Check sheet for the modelled part. Datum: model origin and axes. Units: mm. A direction names the side the tool comes from. Coordinates: 2 decimals unless noted, no trailing zeros. Order: outer loops, then holes, each group sorted by start corner. A loop starts at its lowest first (then second) coordinate and runs counter-clockwise, first axis right, second up.
1. Set-up check for faces 1 (the cylindrical face through (-12.71, -0.95, 3.03)), 2 (the cylindrical face through (0.13, 1.72, -5.45)), 3 (the flat face through (9.525, 2.4, -2.4)): record each of +Z, -Z, +X, -X, +Y, -Y from which the full face is reachable in a straight line by a thin tool's end or side.
2. Thickness scan on line 1 (Y direction, x = 2, z = 0) (3 decimals); line 2 (Z direction, x = 11, y = 0.75); line 3 (Z direction, x = 9, y = -1.25). Record the ranges inside material, lowest first.
3. Cross-section at C-C (x = -12). Enter the section's corners in (y, z) (3 decimals).
4. Draft check along Y on faces 4 (the flat face through (-9.525, 2.4, -2.4)), 5 (the cylindrical face through (-0.221, 0.607, 1.926)), 6 (the cylindrical face through (12.71, -0.95, 3.03)). Enter one of: released by +Y, released by -Y, zero draft, split by the parting line, or undercut.
5. Gauge pin test, flat ends, axial feed: pin 1 Ø2 at (y, z) = (4.5, 1.5) entering from -X (3 decimals); pin 2 Ø4 at (x, z) = (-2.5, 3.5) entering from -Y; pin 3 Ø1 at (x, z) = (-2, -1) entering from +Y. Record the tip position at first contact, or that the pin passes through.
```python
from build123d import *

# Parameters (mm, degrees)
SKETCH34_R                  = 5.715
BOSS_EXTRUDE2_DEPTH         = 15.875
F_21_0_159_DIAMETER_HOLE2_D = 4.0386
SKETCH39_W                  = 6.35
SKETCH39_H                  = 2.54
CHAMFER1_SIZE               = 0.0762
CHAMFER2_SIZE               = 0.0762
CHAMFER8_SIZE               = 0.0762


with BuildPart() as part:
    # Sketch34 → Boss-Extrude2 (new, symmetric)
    with BuildSketch(Plane(origin=(0, 0, 0), x_dir=(0, 0, -1), z_dir=(1, 0, 0))):
        Circle(SKETCH34_R)
    extrude(amount=BOSS_EXTRUDE2_DEPTH, both=True)

    # #21 (0.159) Diameter Hole2 (through all)
    with Locations(Plane(origin=(15.875, 0, 0), x_dir=(0, 0, -1), z_dir=(1, 0, 0))):
        with Locations((0, 0)):
            Hole(F_21_0_159_DIAMETER_HOLE2_D / 2)

    # Sketch39 → Cut-Revolve1 (revolve, cut)
    with BuildSketch(Plane.XY, mode=Mode.PRIVATE) as cut_revolve1_sk:
        with Locations((12.7, 4.445)):
            Rectangle(SKETCH39_W, SKETCH39_H)
    cut_revolve1 = revolve(cut_revolve1_sk.sketch.rotate(Axis((0, 0, 0), (1, 0, 0)), 90), axis=Axis((0, 0, 0), (1, 0, 0)), mode=Mode.SUBTRACT)

    # Chamfer1
    chamfer1_edges = [part.edges().sort_by_distance(p)[0] for p in [
        (15.875, 0, -3.175),
        (9.525, 0, 5.715),
    ]]
    chamfer(chamfer1_edges, length=CHAMFER1_SIZE)

    # Mirror1: Cut-Revolve1 across plane
    add(cut_revolve1.mirror(Plane(origin=(0, 0, 0), x_dir=(0, 0, 1), z_dir=(1, 0, 0))), mode=Mode.SUBTRACT)

    # Chamfer2
    chamfer2_edges = [part.edges().sort_by_distance(p)[0] for p in [
        (-15.875, 0, -3.175),
        (-9.525, 0, 5.715),
    ]]
    chamfer(chamfer2_edges, length=CHAMFER2_SIZE)

    # Chamfer8
    chamfer8_edges = [part.edges().sort_by_distance(p)[0] for p in [
        (15.875, 0, -2.0193),
        (-15.875, 0, -2.0193),
    ]]
    chamfer(chamfer8_edges, length=CHAMFER8_SIZE)


solid = part.part
```
Data:
1. face 1: -X
1. face 2: +X, -X
1. face 3: +X
2. line 1: y = -5.715 to -2.019, 2.019 to 5.715
2. line 2: z = -3.09 to -1.87, 1.87 to 3.09
2. line 3: z = -5.58 to -1.59, 1.59 to 5.58
3. outline: circle Ø6.35 at (0, 0); hole circle Ø4.039 at (0, 0)
4. face 4: zero draft
4. face 5: undercut
4. face 6: split by the parting line
5. pin 1: stops at x = -9.525
5. pin 2: stops at y = -5.51
5. pin 3: stops at y = 5.69
